```python
from build123d import *

# Parameters (mm, degrees)
SKETCH_R       = 6.52296
PAD_DEPTH      = 16
SKETCH001_R    = 3.5
HOLE_DEPTH     = 10
HOLE_TIPS_R    = 3.5
SKETCH002_R    = 3.5
HOLE001_DEPTH  = 8
HOLE001_TIPS_R = 3.5
FILLET_R       = 10
FILLET001_R    = 10
FILLET002_R    = 2
FILLET003_R    = 2
FILLET004_R    = 2
FILLET005_R    = 2


with BuildPart() as part:
    # Sketch → Pad (new body)
    with BuildSketch(Plane.XY):
        Polygon((-100, 0), (0, 0), (0, 7), (-18, 7), (-40, 67), (-60, 67), (-82, 7), (-100, 7), align=None)
        with Locations((-50.016819, 58.031078)):
            Circle(SKETCH_R, mode=Mode.SUBTRACT)
    extrude(amount=PAD_DEPTH)

    # Sketch001 → Hole (cut)
    with BuildSketch(Plane.XZ):
        with Locations((-92.026695, 7.972088)):
            Circle(SKETCH001_R)
    extrude(amount=-HOLE_DEPTH, mode=Mode.SUBTRACT)

    # Hole tips → Hole tip 1 section 0
    with BuildSketch(Plane.XZ.offset(-10), mode=Mode.PRIVATE) as hole_tip_1_s0:
        with Locations((-92.026695, 7.972088)):
            Circle(HOLE_TIPS_R)
    loft([hole_tip_1_s0.sketch, Vertex(-92.026695, 12.103012, 7.972088)], mode=Mode.SUBTRACT)

    # Sketch002 → Hole001 (cut)
    with BuildSketch(Plane.XZ):
        with Locations((-8.022125, 7.974626)):
            Circle(SKETCH002_R)
    extrude(amount=-HOLE001_DEPTH, mode=Mode.SUBTRACT)

    # Hole001 tips → Hole001 tip 1 section 0
    with BuildSketch(Plane.XZ.offset(-8), mode=Mode.PRIVATE) as hole001_tip_1_s0:
        with Locations((-8.022125, 7.974626)):
            Circle(HOLE001_TIPS_R)
    loft([hole001_tip_1_s0.sketch, Vertex(-8.022125, 10.103012, 7.974626)], mode=Mode.SUBTRACT)

    # Fillet
    fillet_edges = [part.edges().sort_by_distance(p)[0] for p in [
        (-40, 67, 8),
    ]]
    fillet(fillet_edges, radius=FILLET_R)

    # Fillet001
    fillet001_edges = [part.edges().sort_by_distance(p)[0] for p in [
        (-60, 67, 8),
    ]]
    fillet(fillet001_edges, radius=FILLET001_R)

    # Fillet002
    fillet002_edges = [part.edges().sort_by_distance(p)[0] for p in [
        (-82, 7, 8),
    ]]
    fillet(fillet002_edges, radius=FILLET002_R)

    # Fillet003
    fillet003_edges = [part.edges().sort_by_distance(p)[0] for p in [
        (-18, 7, 8),
    ]]
    fillet(fillet003_edges, radius=FILLET003_R)

    # Fillet004
    fillet004_edges = [part.edges().sort_by_distance(p)[0] for p in [
        (0, 7, 8),
    ]]
    fillet(fillet004_edges, radius=FILLET004_R)

    # Fillet005
    fillet005_edges = [part.edges().sort_by_distance(p)[0] for p in [
        (-100, 7, 8),
    ]]
    fillet(fillet005_edges, radius=FILLET005_R)


solid = part.part
```
Source: CAD feature listing. Evaluate the final solid. Frame: model axes, mm. A direction names the side the tool comes from. Coordinates: 2 decimals unless noted, no trailing zeros. Loops run counter-clockwise (first coordinate to the right, second up) from the corner with the lowest first, then second, coordinate; pieces in that order, holes last. Notation, with made-up numbers: M -28.75,-3.75 L 1.25,-3.75 A13 cw 1.25,12.25 Z; hole C 60,21.5 d8. An arc over 180 degrees is marked long. Use a Markdown table: item, result. Add a question column.
Q1. First-contact query: pin 1 (7.5 mm diameter, centred on x = -6, z = 9.5, fed in from +Y); pin 2 (1 mm diameter, centred on x = -41, z = 3, fed in from +Y); pin 3 (1.5 mm diameter, centred on x = -43.5, z = 13, fed in from +Y). Flat tips, straight axial feed; report the tip coordinate or a pass-through.
Q2. Draft query along Z for faces 1 (the flat face through (-51, 27, 16)), 2 (the cylindrical face through (-8.478, 3.451, 11.445)), 3 (the cylindrical face through (-88.794, 3.451, 6.632)), 4 (the flat face through (0, 2, 8)). Return one class per face: pulls with the +Z half, pulls with the -Z half, needs draft (parallel to the pull), parting line crosses it, or undercut.
Q3. Section query C-C, the plane z = 14. Return loops of the section in (x, y).
Q4. Material intervals for L1, parallel to X at y = 3.5, z = 7.75; L2, parallel to Y at x = -13.5, z = 13.5; L3, parallel to X at y = 56, z = 9.25, sorted ascending.
Q5. Section query D-D, the plane y = 37. Return loops of the section in (x, z).
Q6. Section query A-A, the plane z = 9. Return loops of the section in (x, y), and give its area (3 significant figures).
Q7. Access query for faces 5 (the flat face through (-87, 7, 8)), 6 (the flat face through (-51, 0, 8)), 7 (the flat face through (-12, 7, 8)). Directions: +Z, -Z, +X, -X, +Y, -Y. A direction counts if a zero-diameter tool reaches every point of the face in a straight line with its end or side. Return the directions, or none.
Q8. Section query B-B, the plane x = -55. Return loops of the section in (y, z).
Result:
| question | item | result |
|---|---|---|
| 1 | pin 1 | stops at y = 7 |
| 1 | pin 2 | stops at y = 65.36 |
| 1 | pin 3 | stops at y = 66.62 |
| 2 | face 1 | pulls with the +Z half |
| 2 | face 2 | undercut |
| 2 | face 3 | undercut |
| 2 | face 4 | needs draft |
| 3 | outline | M -100,0 L 0,0 L 0,5 A2 ccw -2,7 L -16.6,7 A2 cw -18.48,8.31 L -37.6,60.44 A10 ccw -46.98,67 L -53.02,67 A10 ccw -62.4,60.44 L -81.52,8.31 A2 cw -83.4,7 L -98,7 A2 ccw -100,5 Z; hole C -50.02,58.03 d13.05 |
| 4 | L1 | x = -100 to -95.52, -88.53 to -11.51, -4.53 to 0 |
| 4 | L2 | y = 0 to 7 |
| 4 | L3 | x = -64.03 to -56.22, -43.82 to -35.97 |
| 5 | outline | M -71,0 L -29,0 L -29,16 L -71,16 Z |
| 6 | outline | M -100,0 L -95.37,0 L -95.37,7 L -98,7 A2 ccw -100,5 Z; M -88.68,0 L -11.37,0 L -11.37,7 L -16.6,7 A2 cw -18.48,8.31 L -37.6,60.44 A10 ccw -46.98,67 L -53.02,67 A10 ccw -62.4,60.44 L -81.52,8.31 A2 cw -83.4,7 L -88.68,7 Z; M -4.68,0 L 0,0 L 0,5 A2 ccw -2,7 L -4.68,7 Z; hole C -50.02,58.03 d13.05 |
| 6 | area | 2,970 mm2 |
| 7 | face 5 | +Z, -Z, -X, +Y |
| 7 | face 6 | +Z, -Z, +X, -X, -Y |
| 7 | face 7 | +Z, -Z, +X, +Y |
| 8 | outline | M 0,0 L 53.82,0 L 53.82,16 L 0,16 Z; M 62.24,0 L 66.8,0 L 66.8,16 L 62.24,16 Z |
